Read the model definition and answer for the solid it produces. Units are mm, in the model's axes. A direction names the side the tool comes from. Give positions to 0.01 mm unless a question says otherwise; leave off trailing zeros. Write each loop counter-clockwise with the first axis right and the second up, starting at its lowest first coordinate (ties: lowest second). Pieces come first, ordered by that corner, then holes. Notation, with made-up numbers: M 29.25,61.25 L 86.25,61.25 A25 cw 86.25,98.25 Z; hole C -3,-23 d5. An arc over 180 degrees is marked long. Put each result on its own line as item: value.
Autodesk Inventor part; units mm, degrees
ref_plane "YZ Plane" through (0, 0, 0) normal (1, 0, 0) x (0, 1, 0)
ref_plane "XZ Plane" through (0, 0, 0) normal (0, 1, 0) x (-1, 0, 0)
ref_plane "XY Plane" through (0, 0, 0) normal (0, 0, 1) x (1, 0, 0)
sketch "Boceto1" plane through (0, 0, 0) normal (1, 0, 0) x (0, 1, 0)
  line L0 (0, 0) -> (436, 0)
  line L1 (436, 0) -> (436, -531)
  line L2 (436, -531) -> (0, -531)
  line L3 (0, -531) -> (0, 0)
  line L4 (0, -531) -> (12, -531)
  line L5 (12, -531) -> (12, 0)
  line L6 (12, 0) -> (0, 0)
  line L7 (0, 0) -> (0, -531)
  line L8 (436, -531) -> (424, -531)
  line L9 (424, -531) -> (424, -513.995)
  line L10 (436, -513.995) -> (436, -531)
  line L11 (436, 0) -> (424, 0)
  line L12 (424, 0) -> (424, -531)
  line L13 (424, -531) -> (436, -531)
  line L14 (436, -531) -> (436, 0)
  line L15 (0, 0) -> (436, 0)
  line L16 (436, 0) -> (436, -12)
  line L17 (436, -12) -> (0, -12)
  line L18 (0, -12) -> (0, 0)
  line L19 (0, -531) -> (436, -531)
  line L20 (436, -531) -> (436, -519)
  line L21 (436, -519) -> (0, -519)
  line L22 (0, -519) -> (0, -531)
  line L23 (12, -519) -> (147, -519)
  line L24 (147, -519) -> (147, -270)
  line L25 (147, -270) -> (12, -270)
  line L26 (12, -270) -> (12, -519)
  line L27 (12, -270) -> (424, -270)
  line L28 (424, -270) -> (424, -258)
  line L29 (424, -258) -> (12, -258)
  line L30 (12, -258) -> (12, -270)
  line L31 (147, -519) -> (159, -519)
  line L32 (159, -519) -> (159, -12)
  line L33 (159, -12) -> (147, -12)
  line L34 (147, -12) -> (147, -519)
  line L35 (159, -519) -> (283, -519)
  line L36 (283, -519) -> (283, -270)
  line L37 (283, -270) -> (159, -270)
  line L38 (159, -270) -> (159, -519)
  line L39 (283, -519) -> (295, -519)
  line L40 (295, -519) -> (295, -270)
  line L41 (295, -270) -> (283, -270)
  line L42 (283, -270) -> (283, -519)
  line L43 (295, -258) -> (295, -12)
  line L44 (283, -12) -> (283, -258)
  point P0 (424, -12)
  point P1 (159, -258)
  point P2 (159, -270)
  point P3 (12, -12)
  point P4 (147, -258)
  point P5 (424, -519)
  point P6 (424, -519)
  dimension "d0" = 436
  dimension "d1" = 531
  dimension "d2" = 12
  dimension "d3" = 12
  dimension "d4" = 12
  dimension "d5" = 12
  dimension "d6" = 12
  dimension "d7" = 135
  dimension "d8" = 249
  dimension "d9" = 12
  dimension "d10" = 12
  dimension "d11" = 124
  dimension "d12" = 12
extrude "Extrusión2" add sketch "Boceto1" against normal blind 103 contours L0 L5 L17 L3 | L0 L12 L17 L5 | L17 L5 L21 L3 | L0 L1 L17 L12 | L21 L5 L2 L3 | L17 L1 L21 L9 L12 | L29 L34 L25 L5 | L17 L32 L29 L34 | L21 L9 L2 L5 | L12 L27 L32 L29 | L43 L29 L44 L17 | L29 L32 L27 L34 | L24 L27 L32 L21 | L9 L21 L1 L2 | L40 L21 L36 L27
properties part number "Estante"
(1) Section A-A on z = -179.5 is taken. Determine the outline of the cut face in (x, y), and give its area (3 significant figures).
Result:
outline: M -103,0 L 0,0 L 0,12 L -103,12 Z; M -103,147 L 0,147 L 0,159 L -103,159 Z; M -103,283 L 0,283 L 0,295 L -103,295 Z; M -103,424 L 0,424 L 0,436 L -103,436 Z
area: 4,940 mm²
(2) Which of the six approach directions +Z, -Z, +X, -X, +Y, -Y give full straight-line access (tool end or side, diameter ignored) to faces 4 (the face through (-51, 12, -137)), 5 (the face through (-51, 0, -269))?
Result:
face 4: +X, -X
face 5: +Z, -Z, +X, -X, -Y
(3) Straight lines are drawn through the part: line 1 along Y through (x, z) = (-44, -489); line 2 along Z through (x, y) = (-25, 112). For each, find the intervals that lie inside material, in ascending order. Write a range as from..to.
Result:
line 1: y = 0..12, 147..159, 283..295, 424..436
line 2: z = -531..-519, -270..-258, -12..0
(4) Section C-C on x = -13 is taken. Determine the outline of the cut face in (y, z).
Result:
outline: M 0,-531 L 436,-531 L 436,0 L 0,0 Z; hole M 12,-519 L 147,-519 L 147,-270 L 12,-270 Z; hole M 12,-258 L 147,-258 L 147,-12 L 12,-12 Z; hole M 159,-519 L 283,-519 L 283,-270 L 159,-270 Z; hole M 159,-258 L 283,-258 L 283,-12 L 159,-12 Z; hole M 295,-519 L 424,-519 L 424,-270 L 295,-270 Z; hole M 295,-258 L 424,-258 L 424,-12 L 295,-12 Z
(5) For a pull along Y with two mould halves and no side action, classify faces 1 (the face through (-51, 436, -262)), 2 (the face through (-51, 12, -396)), 3 (the face through (0, 201, -264)) as +Y half, -Y half, draft (parallel to the pull), parting line (faces both ways), or undercut.
Result:
face 1: +Y half
face 2: undercut
face 3: draft
(6) Section B-B on y = 176.5 is taken. Determine the outline of the cut face in (x, z).
Result:
outline: M -103,-531 L 0,-531 L 0,-519 L -103,-519 Z; M -103,-270 L 0,-270 L 0,-258 L -103,-258 Z; M -103,-12 L 0,-12 L 0,0 L -103,0 Z
